Geometry check sheet. Reference: the model listing, model coordinates, mm. Face numbers are marked on the shaded views. A direction names the side the tool comes from. Coordinates: 2 decimals unless noted, no trailing zeros. Order: outer loops, then holes, each group sorted by start corner. A loop starts at its lowest first (then second) coordinate and runs counter-clockwise, first axis right, second up. Notation, with made-up numbers: (34, 82) - (70, 82) arc R33 cw to (70, 111) - close; hole circle Ø2 at (-9.75, 31.25). An arc over 180 degrees is marked (long way). Put each result on its own line as item: value.
from build123d import *

# Parameters (mm, degrees)
SKETCH_1_W              = 150
SKETCH_1_H              = 40
EXTRUDE_1_DEPTH         = 20
SKETCH_3_W              = 12
SKETCH_3_H              = 40
EXTRUDE_2_DEPTH         = 40
CUT_EXTRUDE_1_DEPTH     = 40
HOLE_WIZARD_M10_1_D     = 8.5
HOLE_WIZARD_M10_1_DEPTH = 24.5
HOLE_WIZARD_M10_1_TIP   = 2.553657631
SKETCH_7_W              = 16
SKETCH_7_H              = 10
CUT_EXTRUDE_2_DEPTH     = 150


with BuildPart() as part:
    # 草图1 → 凸台-拉伸1 (new body)
    with BuildSketch(Plane(origin=(0, 0, 0), x_dir=(1, 0, 0), z_dir=(0, 1, 0))):
        Rectangle(SKETCH_1_W, SKETCH_1_H)
    extrude(amount=EXTRUDE_1_DEPTH)

    # 草图3 → 凸台-拉伸2 (add)
    with BuildSketch(Plane.XZ):
        with Locations((81, 0)):
            Rectangle(SKETCH_3_W, SKETCH_3_H)
    extrude(amount=-EXTRUDE_2_DEPTH)

    # 草图4 → 切除-拉伸1 (cut)
    with BuildSketch(Plane(origin=(0, 20, 0), x_dir=(1, 0, 0), z_dir=(0, 1, 0))):
        with BuildLine():
            Line((-65, 5.5), (65, 5.5))
            ThreePointArc((65, 5.5), (70.5, 0), (65, -5.5))
            Line((65, -5.5), (-65, -5.5))
            ThreePointArc((-65, -5.5), (-70.5, 0), (-65, 5.5))
        make_face()
    extrude(amount=-CUT_EXTRUDE_1_DEPTH, mode=Mode.SUBTRACT)

    # M10 螺纹孔1
    with Locations(Plane(origin=(87, 0, 0), x_dir=(0, 0, -1), z_dir=(1, 0, 0))):
        with Locations((0, 30)):
            Hole(HOLE_WIZARD_M10_1_D / 2, depth=HOLE_WIZARD_M10_1_DEPTH)
            with Locations((0, 0, -(HOLE_WIZARD_M10_1_DEPTH + HOLE_WIZARD_M10_1_TIP / 2))):  # 118° drill point
                Cone(0, HOLE_WIZARD_M10_1_D / 2, HOLE_WIZARD_M10_1_TIP, mode=Mode.SUBTRACT)

    # 草图7 → 切除-拉伸2 (cut)
    with BuildSketch(Plane.ZY.offset(75)):
        with Locations((0, 5)):
            Rectangle(SKETCH_7_W, SKETCH_7_H)
    extrude(amount=-CUT_EXTRUDE_2_DEPTH, mode=Mode.SUBTRACT)


solid = part.part
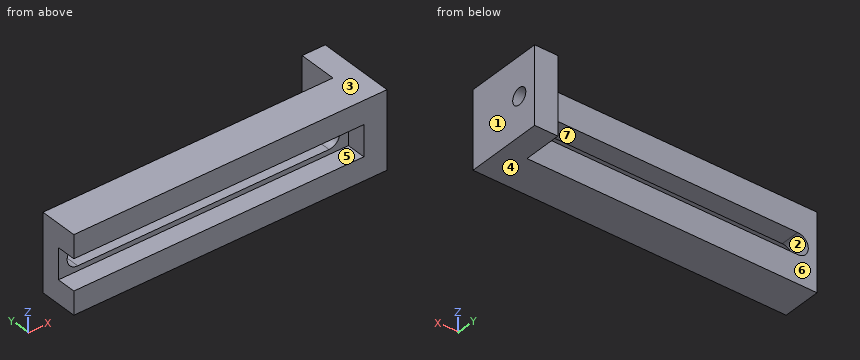
Q1. Depth check by flat-ended pin: pin 1 Ø4 at (x, z) = (-12, -10) entering from +Y; pin 2 Ø17.5 at (x, z) = (-27, -1.5) entering from -Y; pin 3 Ø1 at (x, y) = (0.5, 21.5) entering from -Z; pin 4 Ø2 at (x, z) = (-46.5, -6) entering from -Y. Enter the tip coordinate at first touch or a pass-through.
Answer block:
pin 1: stops at y = 20
pin 2: stops at y = 0
pin 3: passes through
pin 4: stops at y = 10
Q2. Access from +Z, -Z, +X, -X, +Y, -Y to the whole of each face (thin tool, end or side, straight path). Record for the marked faces 5, 6 and 7.
Answer block:
face 5: -X, -Y
face 6: +Z, -Z, -X, +Y
face 7: +Y, -Y
Q3. Thickness scan on L1, parallel to Z at x = -28.5, y = 15.5; L2, parallel to Y at x = 79, z = 0; L3, parallel to Z at x = 44.5, y = 8.5. Record the ranges inside material, lowest first. Write a range as [from, to].
Answer block:
L1: z = [-20, -5.5], [5.5, 20]
L2: y = [0, 25.75], [34.25, 40]
L3: z = [-20, -8], [8, 20]
Q4. Draft check along Z on the marked faces 1, 2, 3 and 4. Enter one of: pulls with the +Z half, pulls with the -Z half, needs draft (parallel to the pull), parting line crosses it, or undercut.
Answer block:
face 1: needs draft
face 2: undercut
face 3: pulls with the +Z half
face 4: pulls with the -Z half
Q5. Section check B-B on x = 62.5. Record the boundary of the cut face in (y, z).
Answer block:
outline: (0, -20) - (20, -20) - (20, -5.5) - (10, -5.5) - (10, -8) - (0, -8) - close; (0, 8) - (10, 8) - (10, 5.5) - (20, 5.5) - (20, 20) - (0, 20) - close
Q6. Section check A-A on z = 0. Record the boundary of the cut face in (x, y), then the cut area to 3 significant figures.
Answer block:
outline: (-75, 10) - (-70.5, 10) - (-70.5, 20) - (-75, 20) - close; (70.5, 10) - (75, 10) - (75, 0) - (87, 0) - (87, 25.75) - (75, 25.75) - (75, 20) - (70.5, 20) - close; (75, 34.25) - (87, 34.25) - (87, 40) - (75, 40) - close
area: 468 mm^2
Q7. Section check D-D on y = 30. Record the boundary of the cut face in (x, z).
Answer block:
outline: (75, -20) - (87, -20) - (87, -4.25) - (75, -4.25) - close; (75, 4.25) - (87, 4.25) - (87, 20) - (75, 20) - close
Q8. Section check C-C on y = 13.5. Record the boundary of the cut face in (x, z).
Answer block:
outline: (-75, -20) - (87, -20) - (87, 20) - (-75, 20) - close; hole (-65, -5.5) - (65, -5.5) arc R5.5 ccw to (65, 5.5) - (-65, 5.5) arc R5.5 ccw to start
